Design review of the part built by this model. Coordinates are the model's own, in mm. Coordinates: 2 decimals unless noted, no trailing zeros. Write each loop counter-clockwise with the first axis right and the second up, starting at its lowest first coordinate (ties: lowest second). Pieces come first, ordered by that corner, then holes. Notation, with made-up numbers: (81.25, -3) -> (99.25, -3) arc R23 cw to (99.25, 23) -> close; hole circle Ø5 at (31, 60). An arc over 180 degrees is marked (long way). One line per question, with ' | ' between items. Start each with the question number.
Q1. Add section B-B on z = -6.5. State the section outline as (x, y) points, and give its area (3 significant figures).
Q2. Wall thickness on probe 1 along X at (y, z) = (1.35, -6.5); probe 2 along X at (y, z) = (1.3, -35); probe 3 along Z at (x, y) = (18, 1.1): over which ranges is each line inside the solid? List them lowest first.
Q3. For P1, Ø1.9, axis at x = 0.5, z = -6, coming from the +Y side; P2, Ø6, axis at x = 20, z = -35, coming from the -Y side, all flat-tipped, find the tip position at first contact; note any pin that passes through.
Q4. Add section A-A on x = 20. State the section outline as (y, z) points.
from build123d import *

# Parameters (mm, degrees)
SKIZZE1_W                       = 60
SKIZZE1_H                       = 60
AUFSATZ_LINEAR_AUSTRAGEN1_DEPTH = 6
BOHRUNG3_D                      = 3.9
BOHRUNG3_CBORE_D                = 6.4
BOHRUNG3_CBORE_DEPTH            = 3.5
BOHRUNG4_D                      = 3.9
BOHRUNG4_DEPTH                  = 100
BOHRUNG4_CBORE_D                = 6.4
BOHRUNG4_CBORE_DEPTH            = 3


with BuildPart() as part:
    # Skizze1 → Aufsatz-Linear austragen1 (new body)
    with BuildSketch(Plane(origin=(0, 0, 0), x_dir=(1, 0, 0), z_dir=(0, 1, 0))):
        with Locations((25, 30)):
            Rectangle(SKIZZE1_W, SKIZZE1_H)
    extrude(amount=AUFSATZ_LINEAR_AUSTRAGEN1_DEPTH)

    # Bohrung3 (through all)
    with Locations(Plane(origin=(20, 0, -25), x_dir=(0, 0, -1), z_dir=(0, -1, 0))):
        with Locations((0, 0), (0, 10), (10, 10), (10, 0)):
            CounterBoreHole(BOHRUNG3_D / 2, BOHRUNG3_CBORE_D / 2, BOHRUNG3_CBORE_DEPTH)

    # Bohrung4
    with Locations(Plane(origin=(1.5, 6, -53.5), x_dir=(0, 0, 1), z_dir=(0, 1, 0))):
        with Locations((0, 0), (0, 47), (47, 47), (47, 0)):
            CounterBoreHole(BOHRUNG4_D / 2, BOHRUNG4_CBORE_D / 2, BOHRUNG4_CBORE_DEPTH, depth=BOHRUNG4_DEPTH)


solid = part.part
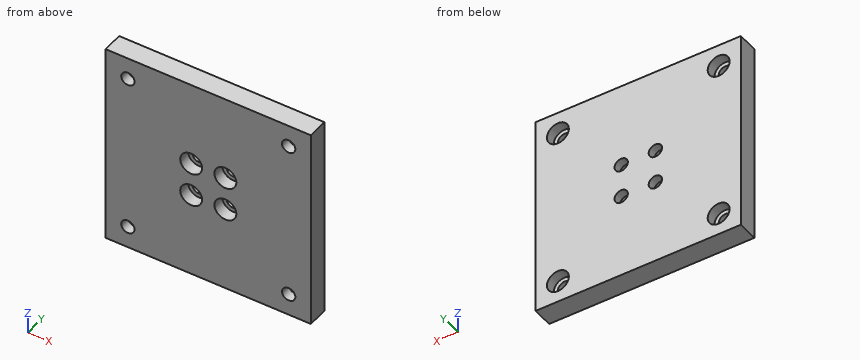
Output values:
1) outline: (-5, 0) -> (-0.45, 0) -> (-0.45, 3) -> (-1.7, 3) -> (-1.7, 6) -> (-5, 6) -> close; (3.45, 0) -> (46.55, 0) -> (46.55, 3) -> (45.3, 3) -> (45.3, 6) -> (4.7, 6) -> (4.7, 3) -> (3.45, 3) -> close; (50.45, 0) -> (55, 0) -> (55, 6) -> (51.7, 6) -> (51.7, 3) -> (50.45, 3) -> close | area: 298 mm2
2) probe 1: x = -5 to -0.45, 3.45 to 46.55, 50.45 to 55 | probe 2: x = -5 to 16.8, 23.2 to 26.8, 33.2 to 55 | probe 3: z = -60 to -37.5, -32.5 to -27.5, -22.5 to 0
3) P1: stops at y = 3 | P2: stops at y = 3.5
4) outline: (0, -60) -> (6, -60) -> (6, -36.95) -> (3.5, -36.95) -> (3.5, -38.2) -> (0, -38.2) -> close; (0, -31.8) -> (3.5, -31.8) -> (3.5, -33.05) -> (6, -33.05) -> (6, -26.95) -> (3.5, -26.95) -> (3.5, -28.2) -> (0, -28.2) -> close; (0, -21.8) -> (3.5, -21.8) -> (3.5, -23.05) -> (6, -23.05) -> (6, 0) -> (0, 0) -> close
